For this review, use the dimensioned drawing (mm, ordinates from the lowest corner) and the shaded views. A direction names the side the tool comes from. Round coordinates to 2 decimals unless told otherwise and drop trailing zeros. Order: outer loops, then holes, each group sorted by start corner. A loop starts at its lowest first (then second) coordinate and runs counter-clockwise, first axis right, second up. Notation, with made-up numbers: M 82.25,37 L 87.25,37 A11 ccw 87.25,54 Z; hole C 16.25,-14 d10. An arc over 180 degrees is marked long. Put each result on its own line as item: value.
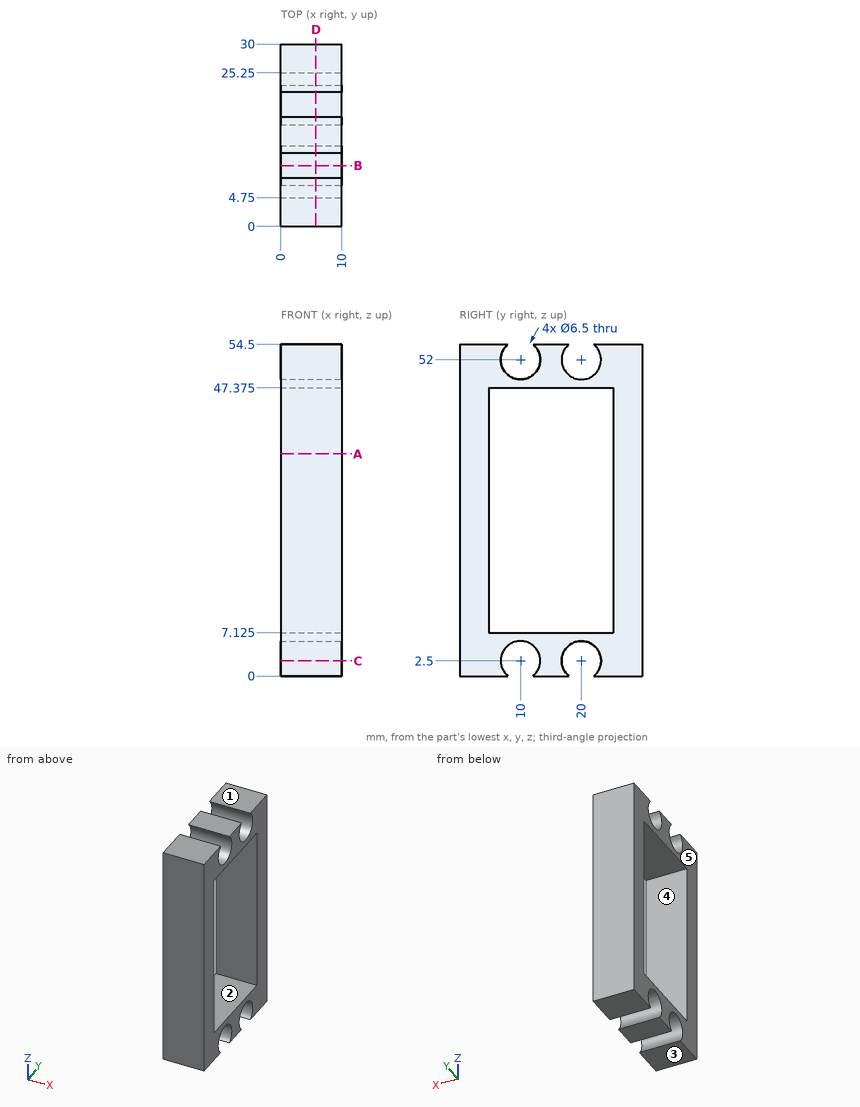
(1) Add section A-A on z = 36.5. Give the boundary of the cut face in (x, y), then the cut area to 3 significant figures.
A:
outline: M 0,0 L 10,0 L 10,4.75 L 0,4.75 Z; M 0,25.25 L 10,25.25 L 10,30 L 0,30 Z
area: 95.0 mm2
(2) Insertion check: pin 1 Ø10.5 at (y, z) = (20, 52) entering from -X; pin 2 Ø8 at (y, z) = (21, 43) entering from +X. Each pin has a flat end and moves straight along its axis. Give the tip position at first contact, or say it passes through.
A:
pin 1: stops at x = 0
pin 2: passes through
(3) Draft analysis for pull direction Z (two halves, no side actions). For the marked faces 1, 2 and 3, state which applies: released by +Z, released by -Z, zero draft, split by the parting line, or undercut.
A:
face 1: released by +Z
face 2: undercut
face 3: released by -Z
(4) Add section B-B on y = 10. Give the boundary of the cut face in (x, z) (3 decimals).
A:
outline: M 0,5.75 L 10,5.75 L 10,7.125 L 0,7.125 Z; M 0,47.375 L 10,47.375 L 10,48.75 L 0,48.75 Z
(5) For the marked faces 4 and 5, list the 3-axis set-ups (+Z, -Z, +X, -X, +Y, -Y) from which the entire face can be reached by the end or side of a thin tool; tool diameter is ignored.
A:
face 4: +X, -X
face 5: +Z, -Z, -X, +Y, -Y
(6) Add section D-D on x = 5.75. Give the boundary of the cut face in (y, z) (3 decimals).
A:
outline: M 0,0 L 7.923,0 A3.25 cw long 12.077,0 L 17.923,0 A3.25 cw long 22.077,0 L 30,0 L 30,54.5 L 22.077,54.5 A3.25 cw long 17.923,54.5 L 12.077,54.5 A3.25 cw long 7.923,54.5 L 0,54.5 Z; hole M 4.75,7.125 L 25.25,7.125 L 25.25,47.375 L 4.75,47.375 Z
(7) To check wall thickness, follow L1, parallel to Y at x = 6, z = 52; L2, parallel to Y at x = 6, z = 45; L3, parallel to Z at x = 6.25, y = 6 (3 decimals). State the ranges of each line that lie inside material, in increasing order.
A:
L1: y = 0 to 6.75, 13.25 to 16.75, 23.25 to 30
L2: y = 0 to 4.75, 25.25 to 30
L3: z = 0 to 7.125, 47.375 to 54.5
(8) Add section C-C on z = 2.5. Give the boundary of the cut face in (x, y).
A:
outline: M 0,0 L 10,0 L 10,6.75 L 0,6.75 Z; M 0,13.25 L 10,13.25 L 10,16.75 L 0,16.75 Z; M 0,23.25 L 10,23.25 L 10,30 L 0,30 Z
